Print and shaded views of the part. All mm, measured from the part's lowest x, y and z. Coordinates: 2 decimals unless noted, no trailing zeros. Use one line per item in the form item = value. Start each with the question number.
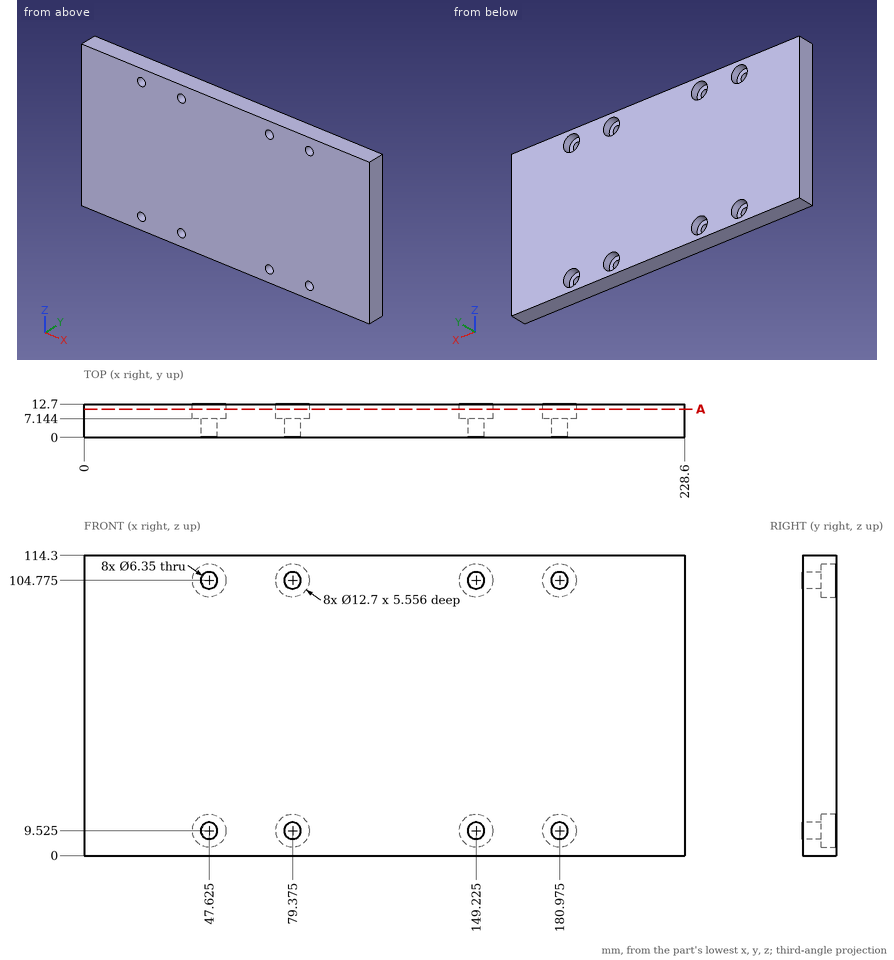
1) Probe L1, parallel to X at y = 4.75, z = 105; L2, parallel to Z at x = 182.5, y = 10.75; L3, parallel to Z at x = 81, y = 3.75. List the from-to ranges inside material, lowest first.
2) Drop a flat-ended pin along its axis: P1, Ø10, axis at x = 149.225, z = 104.775, coming from the +Y side. Give the stop position or say it passes through.
3) Cut at A-A on y = 10.75. Count the separate pieces of the cut face and the enclosed holes in it, then the cut area to 3 significant figures.
Values follow:
q1.L1 = 0 to 44.46, 50.79 to 76.21, 82.54 to 146.06, 152.39 to 177.81, 184.14 to 228.6
q1.L2 = 0 to 3.36, 15.69 to 98.61, 110.94 to 114.3
q1.L3 = 0 to 6.8, 12.25 to 102.05, 107.5 to 114.3
q2.P1 = 7.14
q3.separate_pieces = 1
q3.enclosed_holes = 8
q3.area = 25,100 mm^2
